Autodesk Inventor part; units mm, degrees
ref_plane "YZ Plane" through (0, 0, 0) normal (1, 0, 0) x (0, 1, 0)
ref_plane "XZ Plane" through (0, 0, 0) normal (0, 1, 0) x (-1, 0, 0)
ref_plane "XY Plane" through (0, 0, 0) normal (0, 0, 1) x (1, 0, 0)
sketch "Skizze1" plane through (0, 0, 0) normal (0, 0, 1) x (1, 0, 0)
  line L0 (-17.5, 5) -> (-17.5, 15)
  line L1 (-17.5, 15) -> (-8, 15)
  line L2 (-8, 15) -> (-8, 10)
  line L3 (-8, 10) -> (8, 10)
  line L4 (8, 10) -> (8, 15)
  line L5 (8, 15) -> (17.5, 15)
  line L6 (17.5, 15) -> (17.5, 5)
  line L7 (-7.5, 5) -> (-17.5, 5)
  line L8 (0, 10) -> (0, 0) construction
  line L9 (17.5, 5) -> (7.5, 5)
  line L10 (7.5, 5) -> (7.5, 0)
  line L11 (-7.5, 0) -> (-7.5, 5)
  line L12 (-7.5, 0) -> (7.5, 0)
  point P0 (-12.75, 15)
  dimension "d0" = 16
  dimension "d1" = 5
  dimension "d2" = 35
  dimension "d7" = 15
  dimension "d10" = 5
  dimension "d11" = 15
extrude "Extrusion1" add sketch "Skizze1" along normal blind 10
sketch "Skizze2" plane through (0, 0, 10) normal (0, 0, 1) x (1, 0, 0)
  line L0 (8, 10) -> (-8, 10)
  arc A0 (-6, 10) -> (6, 10) centre (0, 10) ccw
  point P0 (0, 0)
  dimension "d12" = 6
extrude "Extrusion2" cut sketch "Skizze2" against normal blind 10
sketch "Skizze3" plane through (-17.5, 15, 0) normal (0, 1, 0) x (1, 0, 0)
  line L0 (0, 0) -> (0, -10)
  line L1 (35, 0) -> (35, -10)
  line L2 (17.5, 0) -> (17.5, -10) construction
  point P0 (4.75, -5)
  point P1 (30.25, -5)
  point P2 (0, -5)
  point P3 (35, -5)
  dimension "d15" = 25.5
hole "Bohrung1" at (-12.75, 15, 5) at (12.75, 15, 5) direction (0, -1, 0) diameter 4.2 end through all
properties part number "Pleuel_Unterteil" material "Stahl, galvanisiert"
Could you check a few things on this model? Use its own coordinates, in mm. A direction names the side the tool comes from. Coordinates: 2 decimals unless noted, no trailing zeros. Order: outer loops, then holes, each group sorted by start corner. A loop starts at its lowest first (then second) coordinate and runs counter-clockwise, first axis right, second up. Notation, with made-up numbers: (28.25, 68.25) -> (49.25, 68.25) arc R15 ccw to (49.25, 80.25) -> close; hole circle Ø1 at (-24, -30). An arc over 180 degrees is marked (long way). One line per question, with ' | ' between items.
Q1. Imagine slicing it at A-A on y = 14.25. Please give me the cut outline in (x, z).
Return value:
outline: (-17.5, 0) -> (-8, 0) -> (-8, 10) -> (-17.5, 10) -> close; (8, 0) -> (17.5, 0) -> (17.5, 10) -> (8, 10) -> close; hole circle Ø4.2 at (-12.75, 5); hole circle Ø4.2 at (12.75, 5)
Q2. Thinking about a two-plate mould opening in X: for faces 1 (the face through (-15, 15, 5)), 2 (the face through (7, 10, 5)), 3 (the face through (-7.5, 2, 5)), which applies, pulls with the +X half, pulls with the -X half, needs draft (parallel to the pull), parting line crosses it, or undercut?
Return value:
face 1: needs draft | face 2: undercut | face 3: pulls with the -X half
Q3. If I drill on L1, parallel to X at y = 9.75, z = 9.75; L2, parallel to X at y = 10.5, z = 0.5; L3, parallel to Z at x = -12.75, y = 7.5, over which ranges is the centre line in solid material (lowest first)?
Return value:
L1: -17.5 to -5.99, 5.99 to 17.5 | L2: -17.5 to -8, 8 to 17.5 | L3: 0 to 2.9, 7.1 to 10
Q4. I'm going to push flat-ended pins straight in: P1, Ø2, axis at y = 2, z = 4.5, coming from the -X side; P2, Ø1, axis at x = -6.5, z = 3.5, coming from the +Y side. Where does each tip first touch, or does it pass through?
Return value:
P1: x = -7.5 | P2: y = 10
Q5. On a 3-axis mill with a long thin cutter (end or side, diameter ignored), from which of +Z, -Z, +X, -X, +Y, -Y can I reach the whole of each face in a straight line? I mean faces 4 (the face through (-8, 13, 5)), 5 (the face through (7.5, 3, 5)), 6 (the face through (-10, 5, 5)), 7 (the face through (-17.5, 10, 5)). Say none if no direction works.
Return value:
face 4: +Z, -Z, +Y | face 5: +Z, -Z, +X, -Y | face 6: +Z, -Z, -X, -Y | face 7: +Z, -Z, -X, +Y, -Y
Q6. Imagine slicing it at C-C on z = 5. Please give me the cut outline in (x, y), and give its area (3 significant figures).
Return value:
outline: (-17.5, 5) -> (-14.85, 5) -> (-14.85, 15) -> (-17.5, 15) -> close; (-10.65, 5) -> (-7.5, 5) -> (-7.5, 0) -> (7.5, 0) -> (7.5, 5) -> (10.65, 5) -> (10.65, 15) -> (8, 15) -> (8, 10) -> (6, 10) arc R6 cw to (-6, 10) -> (-8, 10) -> (-8, 15) -> (-10.65, 15) -> close; (14.85, 5) -> (17.5, 5) -> (17.5, 15) -> (14.85, 15) -> close | area: 204 mm²
Q7. Imagine slicing it at B-B on x = -12.75. Please give me the cut outline in (y, z), and give its area (3 significant figures).
Return value:
outline: (5, 0) -> (15, 0) -> (15, 2.9) -> (5, 2.9) -> close; (5, 7.1) -> (15, 7.1) -> (15, 10) -> (5, 10) -> close | area: 58.0 mm²
Q8. Imagine slicing it at D-D on z = 8.5. Please give me the cut outline in (x, y), and give its area (3 significant figures).
Return value:
outline: (-17.5, 5) -> (-7.5, 5) -> (-7.5, 0) -> (7.5, 0) -> (7.5, 5) -> (17.5, 5) -> (17.5, 15) -> (8, 15) -> (8, 10) -> (6, 10) arc R6 cw to (-6, 10) -> (-8, 10) -> (-8, 15) -> (-17.5, 15) -> close | area: 288 mm²
